Could you check a few things on this model? Use its own coordinates, in mm. A direction names the side the tool comes from. Round coordinates to 2 decimals unless told otherwise and drop trailing zeros. Write each loop counter-clockwise with the first axis right and the second up, starting at its lowest first coordinate (ties: lowest second). Pieces come first, ordered by that corner, then holes. Notation, with made-up numbers: (-14, 4) -> (23, 4) arc R24 ccw to (23, 26) -> close; hole circle Ø1 at (-14, 34). An arc over 180 degrees is marked (long way). One line per question, with ' | ' between items. Start each with the question number.
1. Imagine slicing it at A-A, the plane z = 5.75. List the corners of the cut face in (x, y) for me (3 decimals), and give its area (3 significant figures).
2. Thinking about a two-plate mould opening in Z: for faces 3 (the cylindrical face through (6.184, -3.56, 4.704)), 4 (the flat face through (0, 0, 4.75)), 5 (the cylindrical face through (1.43, -1.865, -0.912)), which applies, released by +Z, released by -Z, zero draft, split by the parting line, or undercut?
3. For pin 1 Ø4 at (x, z) = (3.5, 4.5) entering from +Y; pin 2 Ø4 at (y, z) = (2, -9.5) entering from +X (3 decimals); pin 3 Ø1.5 at (x, y) = (4.5, 4.5) entering from -Z; pin 4 Ø2 at (x, z) = (-4.5, -9) entering from +Y, each with a flat end and sliding along its axis, tell me the tip position at first contact or that it passes through.
4. For faces 1 (the flat face through (3, -1, 0)), 2 (the cylindrical face through (6.184, 3.56, 4.704)), which set-ups out of +Z, -Z, +X, -X, +Y, -Y let a thin tool reach every point of the face, with its end or its side?
5. Imagine slicing it at D-D, the plane z = -11.25. List the corners of the cut face in (x, y) for me (3 decimals).
6. If I drill on line 1 along Y through (x, z) = (0, 8.4) (3 decimals); line 2 along X through (y, z) = (0, 8.1) (3 decimals); line 3 along Z through (x, y) = (2, 5.5) (3 decimals), over which ranges is the centre line in solid material (lowest first)? Write a range as [from, to].
from build123d import *

# Parameters (mm, degrees)
SKETCH4_R           = 4.7625
BOSS_EXTRUDE1_DEPTH = 9.525
SKETCH5_OUTSIDE_W   = 108.066
SKETCH5_OUTSIDE_H   = 110.03
SKETCH5_OUTSIDE_R   = 6.0325
CUT_EXTRUDE1_DEPTH  = 25.249463052
CUT_EXTRUDE1_DRAFT  = -60
SKETCH6_OUTSIDE_W   = 79.422
SKETCH6_OUTSIDE_H   = 81.386
SKETCH6_OUTSIDE_R   = 6.0325
CUT_EXTRUDE2_DEPTH  = 16.980482888
CUT_EXTRUDE2_DRAFT  = -60
FILLET1_R           = 1.27
SKETCH9_R           = 3.4925
BOSS_EXTRUDE2_DEPTH = 4.7752
SKETCH10_W          = 4.7752
SKETCH10_H          = 3.175


with BuildPart() as part:
    # Sketch3 → Revolve1 (revolve)
    with BuildSketch(Plane(origin=(0, 0, 0), x_dir=(0, 0, -1), z_dir=(1, 0, 0))):
        with BuildLine():
            Line((-4.7498, 2.8575), (-4.7498, 0))
            Line((-4.7498, 0), (12.7, 0))
            Line((12.7, 0), (12.7, 2.8575))
            Line((12.7, 2.8575), (12.3825, 3.175))
            Line((12.3825, 3.175), (2.00025, 3.175))
            Line((2.00025, 3.175), (1.524, 2.350110803))
            Line((1.524, 2.350110803), (0.3175, 2.350110803))
            ThreePointArc((0.3175, 2.350110803), (0.092993597, 2.4431044), (0, 2.667610803))
            Line((0, 2.667610803), (0, 6.35))
            Line((0, 6.35), (-9.525, 6.35))
            Line((-9.525, 6.35), (-9.525, 3.4925))
            Line((-9.525, 3.4925), (-9.2075, 3.175))
            Line((-9.2075, 3.175), (-5.0673, 3.175))
            Line((-5.0673, 3.175), (-4.7498, 2.8575))
        make_face()
    revolve(axis=Axis((0, 0, -12.7), (0, 0, 1)))

    # Sketch4 → Boss-Extrude1 (add)
    with BuildSketch(Plane.XY.offset(9.525)):
        Polygon((-6.35, 3.666174209), (-6.35, -3.666174209), (0, -7.332348419), (6.35, -3.666174209), (6.35, 3.666174209), (0, 7.332348419), align=None)
        Circle(SKETCH4_R, mode=Mode.SUBTRACT)
    extrude(amount=-BOSS_EXTRUDE1_DEPTH)


with BuildPart() as cut_extrude1_tool:
    # Sketch5 outside → Cut-Extrude1 (with draft: the straight prism first)
    with BuildSketch(Plane.XY.offset(9.525)):
        Rectangle(SKETCH5_OUTSIDE_W, SKETCH5_OUTSIDE_H)
        Circle(SKETCH5_OUTSIDE_R, mode=Mode.SUBTRACT)
    extrude(amount=-CUT_EXTRUDE1_DEPTH)
    # Cut-Extrude1: the draft: its side faces are tilted about the plane it starts from
    cut_extrude1_sides = [cut_extrude1_tool.faces().sort_by_distance(p)[0] for p in [
        (0, -55.015, -3.099731526),
        (54.033, 0, -3.099731526),
        (0, 55.015, -3.099731526),
        (-54.033, 0, -3.099731526),
        (-6.0325, 0, -3.099731526),
    ]]
    draft(cut_extrude1_sides, Plane.XY.offset(9.525), CUT_EXTRUDE1_DRAFT)


with BuildPart() as part_1:
    add(part.part)

    # Cut-Extrude1: cut by cut_extrude1_tool
    add(cut_extrude1_tool.part, mode=Mode.SUBTRACT)


with BuildPart() as cut_extrude2_tool:
    # Sketch6 outside → Cut-Extrude2 (with draft: the straight prism first)
    with BuildSketch(Plane(origin=(0, 0, 0), x_dir=(-1, 0, 0), z_dir=(0, 0, -1))):
        Rectangle(SKETCH6_OUTSIDE_W, SKETCH6_OUTSIDE_H)
        Circle(SKETCH6_OUTSIDE_R, mode=Mode.SUBTRACT)
    extrude(amount=-CUT_EXTRUDE2_DEPTH)
    # Cut-Extrude2: the draft: its side faces are tilted about the plane it starts from
    cut_extrude2_sides = [cut_extrude2_tool.faces().sort_by_distance(p)[0] for p in [
        (0, -40.693, 8.490241444),
        (-39.711, 0, 8.490241444),
        (0, 40.693, 8.490241444),
        (39.711, 0, 8.490241444),
        (6.0325, 0, 8.490241444),
    ]]
    draft(cut_extrude2_sides, Plane(origin=(0, 0, 0), x_dir=(-1, 0, 0), z_dir=(0, 0, -1)), CUT_EXTRUDE2_DRAFT)


with BuildPart() as part_2:
    add(part_1.part)

    # Cut-Extrude2: cut by cut_extrude2_tool
    add(cut_extrude2_tool.part, mode=Mode.SUBTRACT)

    # Fillet1
    fillet1_edges = [part_2.edges().sort_by_distance(p)[0] for p in [
        (0, 7.332348419, 4.7625),
        (-6.35, -3.666174209, 4.7625),
        (0, -7.332348419, 4.7625),
        (6.35, -3.666174209, 4.7625),
        (6.35, 3.666174209, 4.7625),
        (-6.35, 3.666174209, 4.7625),
    ]]
    fillet(fillet1_edges, radius=FILLET1_R)

    # Sketch9 → Boss-Extrude2 (add)
    with BuildSketch(Plane.XY.offset(4.7498)):
        Circle(SKETCH9_R)
    extrude(amount=BOSS_EXTRUDE2_DEPTH)


with BuildPart() as body_2:
    # Sketch10 → Revolve2 (revolve)
    with BuildSketch(Plane(origin=(0, 0, 0), x_dir=(0, 0, -1), z_dir=(1, 0, 0))):
        with Locations((-7.1374, 1.5875)):
            Rectangle(SKETCH10_W, SKETCH10_H)
    revolve(axis=Axis((0, 0, -12.7), (0, 0, 1)))


with BuildPart() as part_3:
    add(part_2.part)

    # Combine1: cut body 2
    add(body_2.part, mode=Mode.SUBTRACT)

    # Cut-Extrude3 cone 1 section (through the dimple's axis) → Cut-Extrude3 (revolve, cut)
    with BuildSketch(Plane(origin=(0, 0, 9.525), x_dir=(0, -1, 0), z_dir=(1, 0, 0))):
        Polygon((0, 0), (3.2258, 0), (0, 3.2258), align=None)
    revolve(axis=Axis((0, 0, 9.525), (0, 0, -1)), mode=Mode.SUBTRACT)


solid = part_3.part
Geometry results:
1) outline: (-6.35, -2.933) arc R1.27 ccw to (-5.715, -4.033) -> (-0.635, -6.966) arc R1.27 ccw to (0.635, -6.966) -> (5.715, -4.033) arc R1.27 ccw to (6.35, -2.933) -> (6.35, 2.933) arc R1.27 ccw to (5.715, 4.033) -> (0.635, 6.966) arc R1.27 ccw to (-0.635, 6.966) -> (-5.715, 4.033) arc R1.27 ccw to (-6.35, 2.933) -> close; hole circle Ø6.35 at (0, 0) | area: 107 mm2
2) face 3: zero draft | face 4: released by +Z | face 5: undercut
3) pin 1: stops at y = 6.47 | pin 2: stops at x = 3.175 | pin 3: stops at z = 0 | pin 4: passes through
4) face 1: none | face 2: +Z, -Z, +X, +Y
5) outline: circle Ø6.35 at (0, 0)
6) line 1: y = [-7.136, -3.175], [3.175, 7.136] | line 2: x = [-6.35, -3.175], [3.175, 6.35] | line 3: z = [0, 9.525]
